Geometry: final body of the model. Coordinates: model frame, mm. A direction names the side the tool comes from. Give positions to 0.01 mm unless a question says otherwise; leave off trailing zeros. Order: outer loops, then holes, each group sorted by start corner. A loop starts at its lowest first (then second) coordinate and runs counter-clockwise, first axis right, second up. Notation, with made-up numbers: (27.25, 9) - (36.25, 9) arc R21 cw to (36.25, 37) - close; hole circle Ø5 at (48, 15.5). An arc over 180 degrees is marked (long way). Put each result on its own line as item: value. Start each with the question number.
1. Section A-A on y = -17. Return the cut outline in (x, z).
2. Mould query, pull axis Y, two halves, no side actions, for faces 4 (the cylindrical face through (66.03, -3.62, 5.17)), 5 (the flat face through (47, -19.05, 5)), 6 (the cylindrical face through (3.62, -21.58, 20.03)). Classes: pulls with the +Y half, pulls with the -Y half, needs draft (parallel to the pull), parting line crosses it, or undercut.
3. Set-up query: faces 1 (the cylindrical face through (21.595, -21.778, 25.627)), 2 (the flat face through (34, -18, 0)), 3 (the cylindrical face through (21.595, -3.622, 25.627)). Return all of +Z, -Z, +X, -X, +Y, -Y with unobstructed straight access to the full face (end or side cutting, diameter ignored); none if empty.
4. First-contact query: P1, Ø4, axis at y = -10.5, z = 11, coming from the -X side; P2, Ø5, axis at y = -20.5, z = 35.5, coming from the -X side; P3, Ø7.5, axis at x = 33.5, y = -18.5, coming from the +Z side. Flat tips, straight axial feed; report the tip coordinate or a pass-through.
5. Section B-B on x = 34.5. Return the cut outline in (y, z).
6. Ray query, line 1 along Y through (x, z) = (49, 2.5); line 2 along Z through (x, y) = (37, -22.5); line 3 along Y through (x, z) = (32.5, 2). Return the intervals inside material, ascending. Write a range as from..to.
7. Section D-D on z = 3.5. Count the separate pieces of the cut face and the enclosed holes in it, plus the area to 3 significant figures.
from build123d import *

# Parameters (mm, degrees)
F1_DEPTH = 25.4
F2_R     = 6.35
F3_DEPTH = 50.8
F4_R     = 12.69999
F6_DEPTH = 25.4


# Not quite as in the source:
# - a fillet or chamfer is up to 0.001 mm smaller than in the source, because OpenCascade refuses the exact size


with BuildPart() as f1:
    # F0 (on Front) → F1 (new body)
    with BuildSketch(Plane.XZ):
        Polygon((0, 40.6317008091), (0, 0), (69.85, 0), (69.85, 10.1959701541), (25.413833983, 10.1959701541), (25.413833983, 40.6317008091), align=None)
    extrude(amount=F1_DEPTH)

    # F2 (on face) → F3 (cut)
    with BuildSketch(Plane.XY.offset(40.6317008091)):
        with Locations((12.7069169915, -12.7)):
            Circle(F2_R)
    extrude(amount=-F3_DEPTH, mode=Mode.SUBTRACT)

    # F4 (radius 12.7 in the source; OpenCascade refuses exactly that, so slightly less here)
    f4_edges = [f1.edges().sort_by_distance(p)[0] for p in [
        (25.413834, -25.4, 25.413835),
        (25.413834, 0, 25.413835),
        (0, -25.4, 20.31585),
        (0, 0, 20.31585),
        (69.85, -25.4, 5.097985),
        (69.85, 0, 5.097985),
    ]]
    fillet(f4_edges, radius=F4_R)

    # F5 (on face) → F6 (cut)
    with BuildSketch(Plane.XY.offset(10.1959701541)):
        with BuildLine():
            Line((38.5519873755, -6.3651344446), (37.6653695389, -6.365856045))
            ThreePointArc((37.6653695389, -6.365856045), (31.7677992323, -12.9243723311), (38.113833983, -19.05))
            ThreePointArc((38.113833983, -19.05), (42.6039620435, -17.1901280605), (44.463833983, -12.7))
            ThreePointArc((44.463833983, -12.7), (42.7562888316, -8.3675511568), (38.5519873755, -6.3651344446))
        make_face()
        with BuildLine():
            ThreePointArc((38.5519873755, -6.3651344446), (38.1086658476, -6.3500021031), (37.6653695389, -6.365856045))
            Line((37.6653695389, -6.365856045), (38.5519873755, -6.3651344446))
        make_face()
        with BuildLine():
            ThreePointArc((44.463833983, -12.7), (42.6039620435, -17.1901280605), (38.113833983, -19.05))
            Line((38.113833983, -19.05), (57.15, -19.05))
            ThreePointArc((57.15, -19.05), (50.8000005258, -12.7025840679), (57.1448318647, -6.3500021031))
            Line((57.1448318647, -6.3500021031), (38.5519873755, -6.3651344446))
            ThreePointArc((38.5519873755, -6.3651344446), (42.7562888316, -8.3675511568), (44.463833983, -12.7))
        make_face()
        with BuildLine():
            ThreePointArc((57.1448318647, -6.3500021031), (50.8000005258, -12.7025840679), (57.15, -19.05))
            ThreePointArc((57.15, -19.05), (61.6401280605, -17.1901280605), (63.5, -12.7))
            ThreePointArc((63.5, -12.7), (61.6383004768, -8.2080450993), (57.1448318647, -6.3500021031))
        make_face()
    extrude(amount=-F6_DEPTH, mode=Mode.SUBTRACT)


solid = f1.part
Resolved:
1. outline: (0.75, 0) - (8.03, 0) - (8.03, 40.63) - (0.75, 40.63) - close; (17.38, 0) - (33.44, 0) - (33.44, 10.2) - (24.66, 10.2) - (24.66, 40.63) - (17.38, 40.63) - close; (61.82, 0) - (69.1, 0) - (69.1, 10.2) - (61.82, 10.2) - close
2. face 4: pulls with the +Y half
2. face 5: undercut
2. face 6: pulls with the -Y half
3. face 1: +Z, +X, -Y
3. face 2: -Z, +X, -X, +Y, -Y
3. face 3: +Z, +X, +Y
4. P1: x = 0
4. P2: x = 1.16
4. P3: z = 10.2
5. outline: (-25.4, 0) - (-17.92, 0) - (-17.92, 10.2) - (-25.4, 10.2) - close; (-7.48, 0) - (0, 0) - (0, 10.2) - (-7.48, 10.2) - close
6. line 1: -25.4..-19.05, -6.36..0
6. line 2: 0..10.2
6. line 3: -25.4..-15.67, -9.73..0
7. separate pieces: 1
7. enclosed holes: 2
7. area: 1,140 mm^2
